from build123d import *

# Parameters (mm, degrees)
F0_W      = 57.15
F0_H      = 29.21
F0_R      = 44.45
F1_DEPTH  = 19.05
F2_W      = 19.05
F2_H      = 50.8
F3_DEPTH  = 25.4
F4_W      = 19.05
F4_H      = 50.8
F5_DEPTH  = 25.4
F6_W      = 38.1
F6_H      = 25.4
F6_W_2    = 53.975
F6_H_2    = 19.05
F6_W_3    = 19.05
F6_H_3    = 53.975
F7_DEPTH  = 25.4
F8_R      = 127
F10_DEPTH = 25.4
F11_W     = 6.35
F11_H     = 6.35
F12_DEPTH = 9.525


# Not quite as in the source:
# - a feature names something its author has since deleted; it is built from what else it names


with BuildPart() as f1:
    # F0 (on Top) → F1 (new body)
    with BuildSketch(Plane.XY):
        Polygon((358.775, 0), (0, 0), (0, -889), (152.4, -889), (152.4, -685.8), (254, -685.8), (254, -889), (482.6, -889), (482.6, -685.8), (584.2, -685.8), (584.2, -889), (736.6, -889), (736.6, 0), (377.825, 0), align=None)
        Polygon((152.4, -889), (0, -889), (0, -1143), (358.775, -1143), (377.825, -1143), (736.6, -1143), (736.6, -889), (584.2, -889), (482.6, -889), (254, -889), align=None)
        with Locations((155.575, -1102.995)):
            Rectangle(F0_W, F0_H, mode=Mode.SUBTRACT)
        with Locations((155.575, -929.005)):
            Rectangle(F0_W, F0_H, mode=Mode.SUBTRACT)
        with Locations((368.3, -1022.35)):
            Circle(F0_R, mode=Mode.SUBTRACT)
        with Locations((581.025, -1102.995)):
            Rectangle(F0_W, F0_H, mode=Mode.SUBTRACT)
        with Locations((581.025, -929.005)):
            Rectangle(F0_W, F0_H, mode=Mode.SUBTRACT)
    extrude(amount=F1_DEPTH)

    # F2 (on face) → F3 (cut)
    with BuildSketch(Plane.XY.offset(19.05)):
        with Locations((368.3, -215.9)):
            Rectangle(F2_W, F2_H)
        with Locations((368.3, -393.7)):
            Rectangle(F2_W, F2_H)
        with Locations((368.3, -571.5)):
            Rectangle(F2_W, F2_H)
        with Locations((368.3, -749.3)):
            Rectangle(F2_W, F2_H)
        with Locations((368.3, -927.1)):
            Rectangle(F2_W, F2_H)
    extrude(amount=-F3_DEPTH, mode=Mode.SUBTRACT)

    # F4 (on face) → F5 (cut)
    with BuildSketch(Plane.XY.offset(19.05)):
        with Locations((92.075, -130.9968532642)):
            Rectangle(F4_W, F4_H)
        with Locations((92.075, -257.9968532642)):
            Rectangle(F4_W, F4_H)
        with Locations((644.525, -130.9968532642)):
            Rectangle(F4_W, F4_H)
        with Locations((644.525, -257.9968532642)):
            Rectangle(F4_W, F4_H)
    extrude(amount=-F5_DEPTH, mode=Mode.SUBTRACT)

    # F6 (on face) → F7 (cut)
    with BuildSketch(Plane.XY.offset(19.05)):
        with Locations((311.15, -118.2968532642)):
            Rectangle(F6_W, F6_H)
        with Locations((311.15, -169.0968532642)):
            Rectangle(F6_W, F6_H)
        Polygon((444.5, -170.6843532642), (444.5, -156.3968532642), (406.4, -156.3968532642), (406.4, -181.7968532642), (444.5, -181.7968532642), align=None)
        Polygon((444.5, -116.7093532642), (444.5, -105.5968532642), (406.4, -105.5968532642), (406.4, -130.9968532642), (444.5, -130.9968532642), align=None)
        with Locations((539.75, -99.2468532642)):
            Rectangle(F6_W_2, F6_H_2)
        with Locations((473.075, -143.6968532642)):
            Rectangle(F6_W_3, F6_H_3)
        with Locations((539.75, -188.1468532642)):
            Rectangle(F6_W_2, F6_H_2)
        with Locations((606.425, -143.6968532642)):
            Rectangle(F6_W_3, F6_H_3)
        Polygon((273.05, -207.1968532642), (273.05, -143.6968532642), (273.05, -80.1968532642), (251.5147030354, -80.1968532642), (251.5147030354, -207.1968532642), align=None)
    extrude(amount=-F7_DEPTH, mode=Mode.SUBTRACT)

    # F8
    f8_edges = [f1.edges().sort_by_distance(p)[0] for p in [
        (0, -1143, 9.525),
        (736.6, -1143, 9.525),
    ]]
    fillet(f8_edges, radius=F8_R)

    # F9 (on face) → F10 (cut)
    with BuildSketch(Plane.XY.offset(19.05)):
        Polygon((57.15, -257.9968532642), (38.1, -257.9968532642), (38.1, -273.8015651703), (38.1, -280.3961336613), (38.1, -296.0968532642), (57.15, -296.0968532642), (57.15, -280.3961336613), (57.15, -273.8015651703), align=None)
    extrude(amount=-F10_DEPTH, mode=Mode.SUBTRACT)

    # F11 (on face) → F12 (cut)
    with BuildSketch(Plane(origin=(0, 0, 0), x_dir=(1, 0, 0), z_dir=(0, 0, -1))):
        with Locations((34.925, 277.0468532642)):
            Rectangle(F11_W, F11_H)
        with Locations((60.325, 277.0468532642)):
            Rectangle(F11_W, F11_H)
    extrude(amount=-F12_DEPTH, mode=Mode.SUBTRACT)


solid = f1.part
The model under review builds one solid part; all positions refer to its coordinate system, in mm. Round coordinates to 2 decimals unless told otherwise and drop trailing zeros. Loops run counter-clockwise (first coordinate to the right, second up) from the corner with the lowest first, then second, coordinate; pieces in that order, holes last. Notation, with made-up numbers: (75.25, -14) -> (134.25, -14) arc R18 ccw to (134.25, 0) -> close; hole circle Ø11 at (62.5, 73). An arc over 180 degrees is marked (long way). Write item = value, one per line. Start each with the question number.
Item 1: Insertion check: pin 1 (6 mm diameter, centred on x = 461.5, y = -890, fed in from -Z). The pin has a flat end and moves straight along its axis. Give the tip position at first contact, or say it passes through.
Item 2: To check wall thickness, follow L1, parallel to Y at x = 436, z = 9; L2, parallel to X at y = -259, z = 9; L3, parallel to X at y = -919, z = 9.5 (3 decimals). State the ranges of each line that lie inside material, in increasing order.
Item 3: Take a section at B-B on z = 15. Count the separate pieces of the cut face and the enclosed holes in it, plus the area to 3 significant figures.
Item 4: Mouldability with a two-part tool opening along X and no side actions: class faces 1 (the cylindrical face through (36.215, -1104.81, 9.658)), 2 (the cylindrical face through (392.2, -984.87, 9.39)), 3 (the flat face through (281, -563, 19.05)) as released by +X, released by -X, zero draft, split by the parting line, or undercut.
Item 5: Take a section at A-A on y = -797. Give the boundary of the cut face in (x, z).
Result:
q1.pin_1 = 0
q2.L1 = -1143 to -181.8, -156.4 to -131, -105.6 to 0
q2.L2 = 0 to 38.1, 57.15 to 82.55, 101.6 to 635, 654.05 to 736.6
q2.L3 = 0 to 127, 184.15 to 358.775, 377.825 to 552.45, 609.6 to 736.6
q3.separate_pieces = 1
q3.enclosed_holes = 26
q3.area = 761,000 mm²
q4.face_1 = released by -X
q4.face_2 = undercut
q4.face_3 = zero draft
q5.outline = (0, 0) -> (152.4, 0) -> (152.4, 19.05) -> (0, 19.05) -> close; (254, 0) -> (482.6, 0) -> (482.6, 19.05) -> (254, 19.05) -> close; (584.2, 0) -> (736.6, 0) -> (736.6, 19.05) -> (584.2, 19.05) -> close
